Work out the finished part from the listing and answer in its coordinate system (mm). Face numbers are marked on the shaded views. Coordinates: 2 decimals unless noted, no trailing zeros. Write each loop counter-clockwise with the first axis right and the second up, starting at its lowest first coordinate (ties: lowest second). Pieces come first, ordered by that corner, then holes. Notation, with made-up numbers: M 8.5,66 L 42.5,66 A11 ccw 42.5,77 Z; hole C 78.25,-4.75 d2. An arc over 180 degrees is marked long. Answer as CSV lines item,"result". Start each with the question number.
(1) A cutting plane is placed at B-B on z = 27.5. Give the vertices of the cut face in (x, y) (3 decimals), then the cut area to 4 significant figures.
(2) The mould has two halves that part along X. Classify the marked faces 1, 2 and 3: released by +X, released by -X, zero draft, split by the parting line, or undercut.
(3) Find the intervals of material crossed by L1, parallel to Z at x = -72, y = 4.95; L2, parallel to Z at x = -37, y = 4.75; L3, parallel to X at y = 3.75, z = -24.5 (3 decimals), in increasing order. Write a range as [from, to].
(4) Flat-ended cylindrical pins translate along their axes: P1, Ø0.7, axis at x = -72.5, y = 3.5, coming from the -Z side; P2, Ø7.5, axis at x = 52, z = -46, coming from the +Y side; P3, Ø3.5, axis at x = -73, z = 43.5, coming from the +Y side. Find the tip coordinate at first contact, or state that the pin passes through.
(5) A cutting plane is placed at A-A on x = -59. Give the vertices of the cut face in (y, z).
(6) A cutting plane is placed at C-C on z = -8.92. Give the vertices of the cut face in (x, y) (3 decimals).
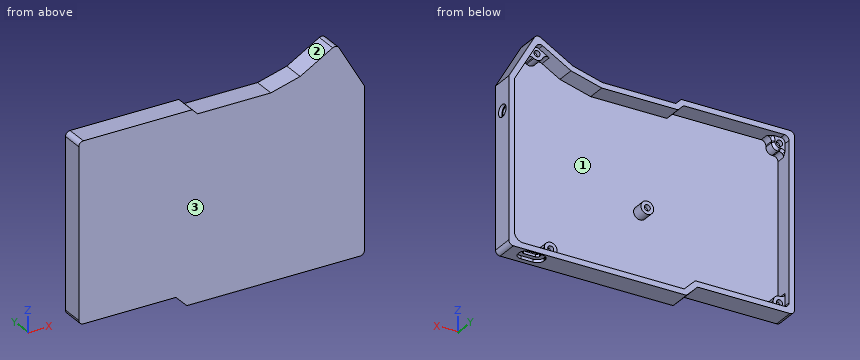
from build123d import *
from OCP.BRepFilletAPI import BRepFilletAPI_MakeChamfer

# Parameters (mm, degrees)
BOSS_EXTRUDE1_DEPTH = 10
BOSS_EXTRUDE2_DEPTH = 2
FILLET1_R           = 2.5
FILLET2_R           = 2.5
FILLET4_R           = 5
SKETCH3_R           = 3.5
BOSS_EXTRUDE3_DEPTH = 6.6
SKETCH5_R           = 1.65
CUT_EXTRUDE1_DEPTH  = 2.5
FILLET3_R           = 2.5
SKETCH6_R           = 2.55
CUT_EXTRUDE2_DEPTH  = 167.136549573
SKETCH7_R           = 3.35
CUT_EXTRUDE3_DEPTH  = 1.8
CUT_EXTRUDE4_REACH  = 141.279
SKETCH8_W           = 9.14
SKETCH8_H           = 3.36
FILLET5_R           = 1.3
CUT_EXTRUDE5_DEPTH  = 1.6
CHAMFER1_SIZE       = 1.5
CHAMFER1_SIZE2      = 1.050311307


with BuildPart() as part:
    # Sketch1 → Boss-Extrude1 (new body)
    with BuildSketch(Plane(origin=(0, 0, 0), x_dir=(1, 0, 0), z_dir=(0, 1, 0))):
        Polygon((78.125, -37.9381301), (62.908489388, -64.283910205), (42.956179643, -52.779359478), (26.916138362, -48.5), (-13.175252532, -48.5), (-16.175252532, -51.5), (-78.125, -51.5), (-78.125, 45.5), (-25.074747468, 45.5), (-19.074747468, 51.5), (78.125, 51.5), align=None)
        Polygon((75.125, -37.134018586), (61.80999823, -60.187537075), (44.11188212, -49.982759925), (27.309448337, -45.5), (-14.417893219, -45.5), (-17.417893219, -48.5), (-75.125, -48.5), (-75.125, 42.5), (-23.832106781, 42.5), (-17.832106781, 48.5), (75.125, 48.5), align=None, mode=Mode.SUBTRACT)
    extrude(amount=BOSS_EXTRUDE1_DEPTH)

    # Sketch2 → Boss-Extrude2 (add)
    with BuildSketch(Plane.XZ):
        Polygon((78.125, -51.5), (78.125, 37.9381301), (62.908489388, 64.283910205), (42.956179643, 52.779359478), (26.916138362, 48.5), (-13.175252532, 48.5), (-16.175252532, 51.5), (-78.125, 51.5), (-78.125, -45.5), (-25.074747468, -45.5), (-19.074747468, -51.5), align=None)
    extrude(amount=BOSS_EXTRUDE2_DEPTH)

    # Fillet1
    fillet1_edges = [part.edges().sort_by_distance(p)[0] for p in [
        (-75.125, 5, -42.5),
        (-75.125, 5, 48.5),
        (61.80999823, 5, 60.187537075),
    ]]
    fillet(fillet1_edges, radius=FILLET1_R)

    # Fillet2
    fillet2_edges = [part.edges().sort_by_distance(p)[0] for p in [
        (62.908489388, 4, 64.283910205),
        (-78.125, 4, 51.5),
        (-78.125, 4, -45.5),
        (78.125, 4, -51.5),
    ]]
    fillet(fillet2_edges, radius=FILLET2_R)

    # Fillet4
    fillet4_edges = [part.edges().sort_by_distance(p)[0] for p in [
        (75.125, 5, -48.5),
    ]]
    fillet(fillet4_edges, radius=FILLET4_R)

    # Sketch3 → Boss-Extrude3 (add)
    with BuildSketch(Plane(origin=(0, 0, 0), x_dir=(1, 0, 0), z_dir=(0, 1, 0))):
        with BuildLine():
            ThreePointArc((-68.5, -45.3), (-69.525126266, -42.825126266), (-72, -41.8))
            ThreePointArc((-72, -41.8), (-73.834848074, -42.319508003), (-75.125, -43.723809973))
            Line((-75.125, -43.723809973), (-75.125, -46))
            ThreePointArc((-75.125, -46), (-74.392766953, -47.767766953), (-72.625, -48.5))
            Line((-72.625, -48.5), (-70.582255312, -48.5))
            ThreePointArc((-70.582255312, -48.5), (-69.066392459, -47.208912464), (-68.5, -45.3))
        make_face()
        with BuildLine():
            Line((-75.125, -46), (-75.125, -43.723809973))
            ThreePointArc((-75.125, -43.723809973), (-74.536075308, -47.712119821), (-70.582255312, -48.5))
            Line((-70.582255312, -48.5), (-72.625, -48.5))
            ThreePointArc((-72.625, -48.5), (-74.392766953, -47.767766953), (-75.125, -46))
        make_face()
        with BuildLine():
            Line((-72, -41.8), (-75.125, -41.8))
            Line((-75.125, -41.8), (-75.125, -43.723809973))
            ThreePointArc((-75.125, -43.723809973), (-73.834848074, -42.319508003), (-72, -41.8))
        make_face()
        with BuildLine():
            ThreePointArc((-70.582255312, 42.5), (-69.066392459, 41.208912464), (-68.5, 39.3))
            Line((-68.5, 39.3), (-68.5, 42.5))
            Line((-68.5, 42.5), (-70.582255312, 42.5))
        make_face()
        with BuildLine():
            ThreePointArc((-72, 35.8), (-69.525126266, 36.825126266), (-68.5, 39.3))
            ThreePointArc((-68.5, 39.3), (-69.066392459, 41.208912464), (-70.582255312, 42.5))
            Line((-70.582255312, 42.5), (-72.625, 42.5))
            ThreePointArc((-72.625, 42.5), (-74.392766953, 41.767766953), (-75.125, 40))
            Line((-75.125, 40), (-75.125, 37.723809973))
            ThreePointArc((-75.125, 37.723809973), (-73.834848074, 36.319508003), (-72, 35.8))
        make_face()
        with BuildLine():
            Line((-72.625, 42.5), (-70.582255312, 42.5))
            ThreePointArc((-70.582255312, 42.5), (-74.536075308, 41.712119821), (-75.125, 37.723809973))
            Line((-75.125, 37.723809973), (-75.125, 40))
            ThreePointArc((-75.125, 40), (-74.392766953, 41.767766953), (-72.625, 42.5))
        make_face()
        with BuildLine():
            Line((-75.125, 35.8), (-72, 35.8))
            ThreePointArc((-72, 35.8), (-73.834848074, 36.319508003), (-75.125, 37.723809973))
            Line((-75.125, 37.723809973), (-75.125, 35.8))
        make_face()
        with Locations(Location((0.325, 8.92, 0), (0, 0, 90))):
            Circle(SKETCH3_R)
        with BuildLine():
            ThreePointArc((54.769807681, 48.5), (53.145, 48.9), (51.520192319, 48.5))
            Line((51.520192319, 48.5), (54.769807681, 48.5))
        make_face()
        with BuildLine():
            Line((54.769807681, 48.5), (51.520192319, 48.5))
            ThreePointArc((51.520192319, 48.5), (50.150269054, 47.21151499), (49.645, 45.4))
            ThreePointArc((49.645, 45.4), (53.145, 41.9), (56.645, 45.4))
            ThreePointArc((56.645, 45.4), (56.139730946, 47.21151499), (54.769807681, 48.5))
        make_face()
        with BuildLine():
            Line((56.645, 48.5), (54.769807681, 48.5))
            ThreePointArc((54.769807681, 48.5), (56.139730946, 47.21151499), (56.645, 45.4))
            Line((56.645, 45.4), (56.645, 48.5))
        make_face()
        with BuildLine():
            Line((51.520192319, 48.5), (49.645, 48.5))
            Line((49.645, 48.5), (49.645, 45.4))
            ThreePointArc((49.645, 45.4), (50.150269054, 47.21151499), (51.520192319, 48.5))
        make_face()
        with BuildLine():
            Line((65.06794725, -54.546742633), (62.39329915, -53.001948322))
            ThreePointArc((62.39329915, -53.001948322), (63.67559788, -54.283168367), (64.145, -56.034018586))
            ThreePointArc((64.145, -56.034018586), (64.144536351, -56.090986384), (64.143145526, -56.14793909))
            Line((64.143145526, -56.14793909), (65.06794725, -54.546742633))
        make_face()
        with BuildLine():
            ThreePointArc((64.145, -56.034018586), (63.67559788, -54.283168367), (62.39329915, -53.001948322))
            ThreePointArc((62.39329915, -53.001948322), (59.73723674, -52.653786957), (57.612929736, -54.285719436))
            ThreePointArc((57.612929736, -54.285719436), (57.145023166, -56.02128423), (57.600288117, -57.760207901))
            Line((57.600288117, -57.760207901), (59.645803824, -58.939657274))
            ThreePointArc((59.645803824, -58.939657274), (61.542115723, -59.188578919), (63.059447202, -58.024248216))
            Line((63.059447202, -58.024248216), (64.143145526, -56.14793909))
            ThreePointArc((64.143145526, -56.14793909), (64.144536351, -56.090986384), (64.145, -56.034018586))
        make_face()
        with BuildLine():
            ThreePointArc((57.600288117, -57.760207901), (61.48240862, -59.432363301), (64.143145526, -56.14793909))
            Line((64.143145526, -56.14793909), (63.059447202, -58.024248216))
            ThreePointArc((63.059447202, -58.024248216), (61.542115723, -59.188578919), (59.645803824, -58.939657274))
            Line((59.645803824, -58.939657274), (57.600288117, -57.760207901))
        make_face()
        with BuildLine():
            Line((57.612929736, -54.285719436), (56.106253452, -56.898743849))
            Line((56.106253452, -56.898743849), (57.600288117, -57.760207901))
            ThreePointArc((57.600288117, -57.760207901), (57.145023166, -56.02128423), (57.612929736, -54.285719436))
        make_face()
        with BuildLine():
            Line((-68.5, -48.5), (-68.5, -45.3))
            ThreePointArc((-68.5, -45.3), (-69.066392459, -47.208912464), (-70.582255312, -48.5))
            Line((-70.582255312, -48.5), (-68.5, -48.5))
        make_face()
    extrude(amount=BOSS_EXTRUDE3_DEPTH)

    # Sketch5 → Cut-Extrude1 (cut)
    with BuildSketch(Plane(origin=(0, 6.6, 0), x_dir=(1, 0, 0), z_dir=(0, 1, 0))):
        with Locations(Location((-72, 39.3, 0), (0, 0, 270))):
            Circle(SKETCH5_R)
        with Locations(Location((0.325, 8.92, 0), (0, 0, 270))):
            Circle(SKETCH5_R)
        with Locations(Location((53.145, 45.4, 0), (0, 0, 270))):
            Circle(SKETCH5_R)
        with Locations(Location((60.645, -56.034018586, 0), (0, 0, 270))):
            Circle(SKETCH5_R)
        with Locations(Location((-72, -45.3, 0), (0, 0, 270))):
            Circle(SKETCH5_R)
    extrude(amount=-CUT_EXTRUDE1_DEPTH, mode=Mode.SUBTRACT)

    # Fillet3
    fillet3_edges = [part.edges().sort_by_distance(p)[0] for p in [
        (-68.5, 3.3, -42.5),
        (-75.125, 3.3, -35.8),
        (56.645, 3.3, -48.5),
        (49.645, 3.3, -48.5),
        (65.06794725, 3.3, 54.546742633),
        (56.106253452, 3.3, 56.898743849),
        (-68.5, 3.3, 48.5),
        (-75.125, 3.3, 41.8),
    ]]
    fillet(fillet3_edges, radius=FILLET3_R)

    # Sketch6 → Cut-Extrude2 (cut, through all)
    with BuildSketch(Plane.ZY.offset(-75.125)):
        with Locations((22.099069046, 4.1)):
            Circle(SKETCH6_R)
    extrude(amount=-CUT_EXTRUDE2_DEPTH, mode=Mode.SUBTRACT)

    # Sketch7 → Cut-Extrude3 (cut)
    with BuildSketch(Plane(origin=(78.125, 0, 0), x_dir=(0, 0, -1), z_dir=(1, 0, 0))):
        with Locations((-22.099069046, 4.1)):
            Circle(SKETCH7_R)
    extrude(amount=-CUT_EXTRUDE3_DEPTH, mode=Mode.SUBTRACT)

    # Sketch8 → Cut-Extrude4 (cut, up to next)
    with BuildSketch(Plane(origin=(0, 0, -51.5), x_dir=(-1, 0, 0), z_dir=(0, 0, -1)), mode=Mode.PRIVATE) as cut_extrude4_sk1:
        with Locations((-62.66, 5.02)):
            Rectangle(SKETCH8_W, SKETCH8_H)
    cut_extrude4_tool1 = extrude(cut_extrude4_sk1.sketch, amount=-CUT_EXTRUDE4_REACH, mode=Mode.PRIVATE) & part.part
    add(cut_extrude4_tool1.solids().sort_by_distance((62.66, 5.02, -51.5))[0], mode=Mode.SUBTRACT)

    # Fillet5
    fillet5_edges = [part.edges().sort_by_distance(p)[0] for p in [
        (67.23, 3.34, -50),
        (58.09, 3.34, -49.883244788),
        (58.09, 6.7, -50),
        (67.23, 6.7, -50),
    ]]
    fillet(fillet5_edges, radius=FILLET5_R)

    # Sketch9 → Cut-Extrude5 (cut)
    with BuildSketch(Plane(origin=(0, 0, -51.5), x_dir=(-1, 0, 0), z_dir=(0, 0, -1))):
        with BuildLine():
            Line((-69.73, 5.4), (-69.73, 4.64))
            ThreePointArc((-69.73, 4.64), (-68.617005769, 1.952994231), (-65.93, 0.84))
            Line((-65.93, 0.84), (-59.39, 0.84))
            ThreePointArc((-59.39, 0.84), (-56.702994231, 1.952994231), (-55.59, 4.64))
            Line((-55.59, 4.64), (-55.59, 5.4))
            ThreePointArc((-55.59, 5.4), (-56.702994231, 8.087005769), (-59.39, 9.2))
            Line((-59.39, 9.2), (-65.93, 9.2))
            ThreePointArc((-65.93, 9.2), (-68.617005769, 8.087005769), (-69.73, 5.4))
        make_face()
    extrude(amount=-CUT_EXTRUDE5_DEPTH, mode=Mode.SUBTRACT)

    # Chamfer1: one chamfer whose edges measure the first distance from different faces: ONE call of the kernel's chamfer builder (chamfer() names one face for all edges)
    chamfer1_edges_1 = [part.edges().sort_by_distance(p)[0] for p in [
        (-68.5, 6.6, 45.65),
    ]]
    chamfer1_side_1 = [part.faces().sort_by_distance(p)[0] for p in [
        (-68.5, 3.3, 45.65),
    ]]
    chamfer1_edges_2 = [part.edges().sort_by_distance(p)[0] for p in [
        (-69.525126266, 6.6, 42.825126266),
    ]]
    chamfer1_side_2 = [part.faces().sort_by_distance(p)[0] for p in [
        (-69.525126266, 3.3, 42.825126266),
    ]]
    chamfer1_edges_3 = [part.edges().sort_by_distance(p)[0] for p in [
        (-72.3125, 6.6, 41.8),
    ]]
    chamfer1_side_3 = [part.faces().sort_by_distance(p)[0] for p in [
        (-72.3125, 3.3, 41.8),
    ]]
    chamfer1_edges_4 = [part.edges().sort_by_distance(p)[0] for p in [
        (-67.767766953, 6.6, 47.767766953),
    ]]
    chamfer1_side_4 = [part.faces().sort_by_distance(p)[0] for p in [
        (-67.767766953, 3.3, 47.767766953),
    ]]
    chamfer1_edges_5 = [part.edges().sort_by_distance(p)[0] for p in [
        (-74.392766953, 6.6, 41.067766953),
    ]]
    chamfer1_side_5 = [part.faces().sort_by_distance(p)[0] for p in [
        (-74.392766953, 3.3, 41.067766953),
    ]]
    chamfer1 = BRepFilletAPI_MakeChamfer(part.part.solid().wrapped)
    for e in chamfer1_edges_1:
        chamfer1.Add(CHAMFER1_SIZE, CHAMFER1_SIZE2, e.wrapped, chamfer1_side_1[0].wrapped)  # the first distance lies on this face
    for e in chamfer1_edges_2:
        chamfer1.Add(CHAMFER1_SIZE, CHAMFER1_SIZE2, e.wrapped, chamfer1_side_2[0].wrapped)  # the first distance lies on this face
    for e in chamfer1_edges_3:
        chamfer1.Add(CHAMFER1_SIZE, CHAMFER1_SIZE2, e.wrapped, chamfer1_side_3[0].wrapped)  # the first distance lies on this face
    for e in chamfer1_edges_4:
        chamfer1.Add(CHAMFER1_SIZE, CHAMFER1_SIZE2, e.wrapped, chamfer1_side_4[0].wrapped)  # the first distance lies on this face
    for e in chamfer1_edges_5:
        chamfer1.Add(CHAMFER1_SIZE, CHAMFER1_SIZE2, e.wrapped, chamfer1_side_5[0].wrapped)  # the first distance lies on this face
    add(Compound.cast(chamfer1.Shape()), mode=Mode.REPLACE)


solid = part.part
Here are the results:
1,outline,"M -78.125,-2 L 78.125,-2 L 78.125,10 L 75.125,10 L 75.125,0 L -75.125,0 L -75.125,10 L -78.125,10 Z"
1,area,"372.5 mm^2"
2,face 1,"undercut"
2,face 2,"released by -X"
2,face 3,"zero draft"
3,L1,"z = [-45.5, -40.95], [-37.65, -35.8], [41.8, 43.65], [46.95, 51.5]"
3,L2,"z = [-45.5, -42.5], [48.5, 51.5]"
3,L3,"x = [-78.125, -75.125], [75.125, 78.125]"
4,P1,"stops at z = -45.5"
4,P2,"stops at y = 10"
4,P3,"stops at y = 6.6"
5,outline,"M -2,-45.5 L 10,-45.5 L 10,-42.5 L 0,-42.5 L 0,48.5 L 10,48.5 L 10,51.5 L -2,51.5 Z"
6,outline,"M -78.125,-2 L 78.125,-2 L 78.125,10 L 75.125,10 L 75.125,0 L 3.825,0 L 3.825,6.6 L 1.975,6.6 L 1.975,4.1 L -1.325,4.1 L -1.325,6.6 L -3.175,6.6 L -3.175,0 L -75.125,0 L -75.125,10 L -78.125,10 Z"
